from build123d import *

# Parameters (mm, degrees)
F1_DEPTH = 38
F2_R     = 5
F3_R     = 2.2
F3_R_2   = 1.75
F4_DEPTH = 10.001


with BuildPart() as f1:
    # F0 (on Front) → F1 (new body)
    with BuildSketch(Plane.XZ):
        Polygon((-11, 10), (-11, 0), (11, 0), (11, 10), (5, 10), (0, 5), (-5, 10), align=None)
    extrude(amount=-F1_DEPTH)

    # F2
    f2_edges = [f1.edges().sort_by_distance(p)[0] for p in [
        (11, 38, 5),
        (-11, 38, 5),
    ]]
    fillet(f2_edges, radius=F2_R)

    # F3 (on Top) → F4 (cut, through all)
    with BuildSketch(Plane.XY):
        with Locations((0, 6.5)):
            Circle(F3_R)
        with Locations((0, 22.5)):
            Circle(F3_R)
        with Locations((0, 14.5)):
            Circle(F3_R_2)
    extrude(amount=F4_DEPTH, mode=Mode.SUBTRACT)


solid = f1.part
Here's how the part is built. I have some questions about the finished solid (model axes, mm). A direction names the side the tool comes from. Round coordinates to 2 decimals unless told otherwise and drop trailing zeros. Order: outer loops, then holes, each group sorted by start corner. A loop starts at its lowest first (then second) coordinate and runs counter-clockwise, first axis right, second up. Notation, with made-up numbers: M 42.25,23.25 L 82.25,23.25 A11 cw 82.25,38.25 Z; hole C 3.5,31 d1. An arc over 180 degrees is marked long. Return JSON: item names as keys, results as strings. Group by question number.
1. If we mould it in two halves opening along Y, with no side actions, what happens to faces 3 (the face through (0, 0, 4)), 4 (the face through (-8, 19, 10)), 5 (the face through (2.1, 7.16, 3.55))? For each: pulls with the +Y half, pulls with the -Y half, needs draft (parallel to the pull), parting line crosses it, or undercut.
2. If we section it at C-C on z = 1: List the corners of the cut face in (x, y) for me, then the cut area to 3 significant figures.
3. If we section it at B-B on z = 8.75: List the corners of the cut face in (x, y) for me.
4. If we section it at A-A on y = 14.5: List the corners of the cut face in (x, z) for me, then the cut area to 3 significant figures.
5. Please list where these lines run through material, in increasing order: probe 1 along Y at (x, z) = (0, 3.75); probe 2 along X at (y, z) = (14.5, 4.25); probe 3 along X at (y, z) = (22.5, 4.5).
6. If we section it at D-D on x = -1: List the corners of the cut face in (y, z) for me, then the cut area to 3 significant figures.
7. On a 3-axis mill with a long thin cutter (end or side, diameter ignored), from which of +Z, -Z, +X, -X, +Y, -Y can I reach the whole of each face in a straight line? I mean faces 1 (the face through (2.032, 21.657, 3.55)), 2 (the face through (3, 19, 8)). Say none if no direction works.
Reply:
{
 "1": {"face 3": "pulls with the -Y half", "face 4": "needs draft", "face 5": "undercut"},
 "2": {"outline": "M -11,0 L 11,0 L 11,33 A5 ccw 6,38 L -6,38 A5 ccw -11,33 Z; hole C 0,6.5 d4.4; hole C 0,22.5 d4.4; hole C 0,14.5 d3.5", "area": "785 mm^2"},
 "3": {"outline": "M -11,0 L -3.75,0 L -3.75,38 L -6,38 A5 ccw -11,33 Z; M 3.75,0 L 11,0 L 11,33 A5 ccw 6,38 L 3.75,38 Z"},
 "4": {"outline": "M -11,0 L -1.75,0 L -1.75,6.75 L -5,10 L -11,10 Z; M 1.75,0 L 11,0 L 11,10 L 5,10 L 1.75,6.75 Z", "area": "174 mm^2"},
 "5": {"probe 1": "0 to 4.3, 8.7 to 12.75, 16.25 to 20.3, 24.7 to 38", "probe 2": "-11 to -1.75, 1.75 to 11", "probe 3": "-11 to -2.2, 2.2 to 11"},
 "6": {"outline": "M 0,0 L 4.54,0 L 4.54,6 L 0,6 Z; M 8.46,0 L 13.06,0 L 13.06,6 L 8.46,6 Z; M 15.94,0 L 20.54,0 L 20.54,6 L 15.94,6 Z; M 24.46,0 L 38,0 L 38,6 L 24.46,6 Z", "area": "164 mm^2"},
 "7": {"face 1": "+Z, -Z", "face 2": "+Z, +Y, -Y"}
}
